Design review of the part built by this model. Coordinates are the model's own, in mm. Face numbers are marked on the shaded views. A direction names the side the tool comes from. Coordinates: 2 decimals unless noted, no trailing zeros. Loops run counter-clockwise (first coordinate to the right, second up) from the corner with the lowest first, then second, coordinate; pieces in that order, holes last.
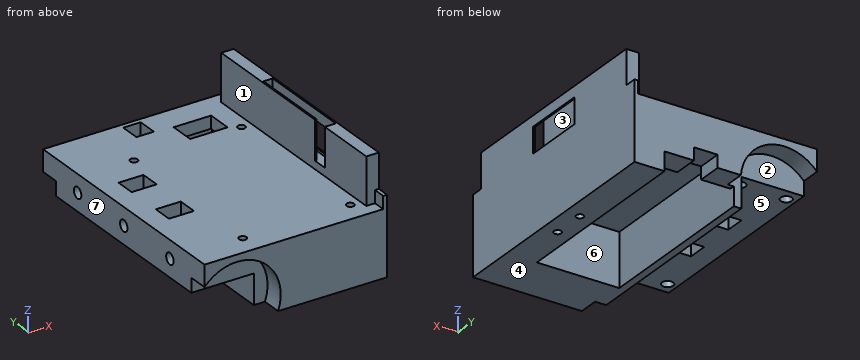
from build123d import *

# Parameters (mm, degrees)
SKETCH1_W           = 72
SKETCH1_H           = 26.25
BOSS_EXTRUDE1_DEPTH = 98
SKETCH3_W           = 24
SKETCH3_H           = 12
CUT_EXTRUDE2_DEPTH  = 98
SKETCH4_W           = 1
SKETCH4_H           = 14.25
BOSS_EXTRUDE2_DEPTH = 98
SKETCH8_R           = 17.5
CUT_EXTRUDE6_DEPTH  = 8
CUT_EXTRUDE7_START  = -8
SKETCH9_R           = 17.5
CUT_EXTRUDE7_DEPTH  = 8
SKETCH10_R          = 2.25
CUT_EXTRUDE8_DEPTH  = 4.25
SKETCH11_W          = 33
SKETCH11_H          = 67.5
CUT_EXTRUDE9_DEPTH  = 21.25
SKETCH12_W          = 33
SKETCH12_H          = 7.5
CUT_EXTRUDE10_DEPTH = 21.25
SKETCH13_W          = 9.5
SKETCH13_H          = 10
CUT_EXTRUDE11_DEPTH = 21.25
SKETCH14_W          = 5
SKETCH14_H          = 5
CUT_EXTRUDE13_DEPTH = 101.25
SKETCH17_W          = 7
SKETCH17_H          = 8
CUT_EXTRUDE14_DEPTH = 7
SKETCH18_W          = 5.398243629
SKETCH18_H          = 5.439982626
BOSS_EXTRUDE3_DEPTH = 2
SKETCH19_W          = 15
SKETCH19_H          = 15
CUT_EXTRUDE15_DEPTH = 12
SKETCH20_W          = 15.253773686
SKETCH20_H          = 5.298590198
BOSS_EXTRUDE5_DEPTH = 5
SKETCH22_R          = 1.5
CUT_EXTRUDE16_DEPTH = 8.2
SKETCH23_W          = 10
SKETCH23_H          = 8
CUT_EXTRUDE18_DEPTH = 125.988249448
SKETCH25_R          = 2.25
CUT_EXTRUDE20_DEPTH = 6.25
SKETCH26_W          = 7
SKETCH26_H          = 8
CUT_EXTRUDE21_DEPTH = 124.057913195
SKETCH28_W          = 7.366793482
SKETCH28_H          = 8.135980894
BOSS_EXTRUDE6_DEPTH = 2
SKETCH31_R          = 1.5
CUT_EXTRUDE24_DEPTH = 3.25
SKETCH32_W          = 5
SKETCH32_H          = 98
BOSS_EXTRUDE7_DEPTH = 18.75
SKETCH34_W          = 5
SKETCH34_H          = 5
CUT_EXTRUDE27_DEPTH = 13.75
SKETCH35_W          = 3.5
SKETCH35_H          = 5
CUT_EXTRUDE28_DEPTH = 5
SKETCH37_W          = 10.25
SKETCH37_H          = 25.25
CUT_EXTRUDE29_DEPTH = 3
SKETCH36_W          = 3.65
SKETCH36_H          = 38.25
CUT_EXTRUDE30_DEPTH = 15.5
SKETCH38_W          = 0.68
SKETCH38_H          = 6
CUT_EXTRUDE31_DEPTH = 15.5


with BuildPart() as part:
    # Sketch1 → Boss-Extrude1 (new body)
    with BuildSketch(Plane(origin=(0, 0, 0), x_dir=(1, 0, 0), z_dir=(0, 1, 0))):
        with Locations((-36, -13.125)):
            Rectangle(SKETCH1_W, SKETCH1_H)
    extrude(amount=BOSS_EXTRUDE1_DEPTH)

    # Sketch3 → Cut-Extrude2 (cut)
    with BuildSketch(Plane.XZ):
        with Locations((-60, 6)):
            Rectangle(SKETCH3_W, SKETCH3_H)
    extrude(amount=-CUT_EXTRUDE2_DEPTH, mode=Mode.SUBTRACT)

    # Sketch4 → Boss-Extrude2 (add)
    with BuildSketch(Plane(origin=(0, 0, 0), x_dir=(-1, 0, 0), z_dir=(0, -1, 0))):
        with Locations((72.5, -19.125)):
            Rectangle(SKETCH4_W, SKETCH4_H)
    extrude(amount=-BOSS_EXTRUDE2_DEPTH)

    # Sketch8 → Cut-Extrude6 (cut)
    with BuildSketch(Plane.XZ):
        with Locations((-60, 6)):
            Circle(SKETCH8_R)
    extrude(amount=-CUT_EXTRUDE6_DEPTH, mode=Mode.SUBTRACT)

    # Sketch9 → Cut-Extrude7 (cut)
    with BuildSketch(Plane(origin=(0, 98, 0), x_dir=(1, 0, 0), z_dir=(0, 1, 0)).offset(CUT_EXTRUDE7_START)):
        with Locations((-60, -6)):
            Circle(SKETCH9_R)
    extrude(amount=CUT_EXTRUDE7_DEPTH, mode=Mode.SUBTRACT)

    # Sketch10 → Cut-Extrude8 (cut)
    with BuildSketch(Plane(origin=(0, 0, 12), x_dir=(-1, 0, 0), z_dir=(0, 0, -1))):
        with Locations((69.25, 85)):
            Circle(SKETCH10_R)
        with Locations((50.75, 85)):
            Circle(SKETCH10_R)
        with Locations((69.25, 13)):
            Circle(SKETCH10_R)
        with Locations((50.75, 13)):
            Circle(SKETCH10_R)
    extrude(amount=-CUT_EXTRUDE8_DEPTH, mode=Mode.SUBTRACT)

    # Sketch11 → Cut-Extrude9 (cut)
    with BuildSketch(Plane(origin=(0, 0, 0), x_dir=(-1, 0, 0), z_dir=(0, 0, -1))):
        with Locations((28.5, 54.25)):
            Rectangle(SKETCH11_W, SKETCH11_H)
    extrude(amount=-CUT_EXTRUDE9_DEPTH, mode=Mode.SUBTRACT)

    # Sketch12 → Cut-Extrude10 (cut)
    with BuildSketch(Plane(origin=(0, 98, 0), x_dir=(1, 0, 0), z_dir=(0, 1, 0))):
        with Locations((-28.5, -3.75)):
            Rectangle(SKETCH12_W, SKETCH12_H)
    extrude(amount=-CUT_EXTRUDE10_DEPTH, mode=Mode.SUBTRACT)

    # Sketch13 → Cut-Extrude11 (cut)
    with BuildSketch(Plane(origin=(0, 98, 0), x_dir=(1, 0, 0), z_dir=(0, 1, 0))):
        with Locations((-28.5, -7.5)):
            Rectangle(SKETCH13_W, SKETCH13_H)
    extrude(amount=-CUT_EXTRUDE11_DEPTH, mode=Mode.SUBTRACT)

    # Sketch14 → Cut-Extrude13 (cut)
    with BuildSketch(Plane(origin=(0, 20.5, 0), x_dir=(1, 0, 0), z_dir=(0, 1, 0))):
        with Locations((-39.5, -12)):
            Rectangle(SKETCH14_W, SKETCH14_H)
    extrude(amount=CUT_EXTRUDE13_DEPTH, mode=Mode.SUBTRACT)

    # Sketch17 → Cut-Extrude14 (cut)
    with BuildSketch(Plane(origin=(0, 0, 7.5), x_dir=(-1, 0, 0), z_dir=(0, 0, -1))):
        with Locations((38.75, 92)):
            Rectangle(SKETCH17_W, SKETCH17_H)
    extrude(amount=-CUT_EXTRUDE14_DEPTH, mode=Mode.SUBTRACT)

    # Sketch18 → Boss-Extrude3 (add)
    with BuildSketch(Plane(origin=(0, 98, 0), x_dir=(1, 0, 0), z_dir=(0, 1, 0))):
        with Locations((-39.480706385, -11.994977786)):
            Rectangle(SKETCH18_W, SKETCH18_H)
    extrude(amount=-BOSS_EXTRUDE3_DEPTH)

    # Sketch19 → Cut-Extrude15 (cut)
    with BuildSketch(Plane.XY.offset(26.25)):
        with Locations((-20.5, 79.5)):
            Rectangle(SKETCH19_W, SKETCH19_H)
    extrude(amount=-CUT_EXTRUDE15_DEPTH, mode=Mode.SUBTRACT)

    # Sketch20 → Boss-Extrude5 (add)
    with BuildSketch(Plane.XY.offset(26.25)):
        with Locations((-20.373113157, 74.350704901)):
            Rectangle(SKETCH20_W, SKETCH20_H)
    extrude(amount=-BOSS_EXTRUDE5_DEPTH)

    # Sketch22 → Cut-Extrude16 (cut)
    with BuildSketch(Plane(origin=(0, 0, 0), x_dir=(-1, 0, 0), z_dir=(0, 0, -1))):
        with Locations((6, 55.73)):
            Circle(SKETCH22_R)
        with Locations((6, 42.27)):
            Circle(SKETCH22_R)
    extrude(amount=-CUT_EXTRUDE16_DEPTH, mode=Mode.SUBTRACT)

    # Sketch23 → Cut-Extrude18 (cut, through all)
    with BuildSketch(Plane.XY.offset(26.25)):
        with Locations((-60, 37.7)):
            Rectangle(SKETCH23_W, SKETCH23_H)
        with Locations((-60, 60.3)):
            Rectangle(SKETCH23_W, SKETCH23_H)
    extrude(amount=-CUT_EXTRUDE18_DEPTH, mode=Mode.SUBTRACT)

    # Sketch25 → Cut-Extrude20 (cut)
    with BuildSketch(Plane.ZY.offset(73)):
        with Locations((19.125, 77)):
            Circle(SKETCH25_R)
        with Locations((19.125, 49)):
            Circle(SKETCH25_R)
        with Locations((19.125, 21)):
            Circle(SKETCH25_R)
    extrude(amount=-CUT_EXTRUDE20_DEPTH, mode=Mode.SUBTRACT)

    # Sketch26 → Cut-Extrude21 (cut, through all)
    with BuildSketch(Plane(origin=(0, 0, 14.5), x_dir=(-1, 0, 0), z_dir=(0, 0, -1))):
        with Locations((38.75, 92)):
            Rectangle(SKETCH26_W, SKETCH26_H)
    extrude(amount=-CUT_EXTRUDE21_DEPTH, mode=Mode.SUBTRACT)

    # Sketch28 → Boss-Extrude6 (add)
    with BuildSketch(Plane(origin=(0, 0, 7.5), x_dir=(-1, 0, 0), z_dir=(0, 0, -1))):
        with Locations((38.749742444, 92.067990447)):
            Rectangle(SKETCH28_W, SKETCH28_H)
    extrude(amount=-BOSS_EXTRUDE6_DEPTH)

    # Sketch31 → Cut-Extrude24 (cut)
    with BuildSketch(Plane.XY.offset(26.25)):
        with Locations((-52.007752906, 74.651528785)):
            Circle(SKETCH31_R)
        with Locations((-9.007752906, 74.651528785)):
            Circle(SKETCH31_R)
        with Locations((-9.007752906, 8.625682812)):
            Circle(SKETCH31_R)
        with Locations((-52.007752906, 8.625682812)):
            Circle(SKETCH31_R)
    extrude(amount=-CUT_EXTRUDE24_DEPTH, mode=Mode.SUBTRACT)

    # Sketch32 → Boss-Extrude7 (add)
    with BuildSketch(Plane.XY.offset(26.25)):
        with Locations((-2.5, 49)):
            Rectangle(SKETCH32_W, SKETCH32_H)
    extrude(amount=BOSS_EXTRUDE7_DEPTH)

    # Sketch34 → Cut-Extrude27 (cut)
    with BuildSketch(Plane.XY.offset(45)):
        with Locations((-2.5, 95.5)):
            Rectangle(SKETCH34_W, SKETCH34_H)
        with Locations((-2.5, 2.5)):
            Rectangle(SKETCH34_W, SKETCH34_H)
    extrude(amount=-CUT_EXTRUDE27_DEPTH, mode=Mode.SUBTRACT)

    # Sketch35 → Cut-Extrude28 (cut)
    with BuildSketch(Plane.XY.offset(31.25)):
        with Locations((-3.25, 95.5)):
            Rectangle(SKETCH35_W, SKETCH35_H)
        with Locations((-3.25, 2.5)):
            Rectangle(SKETCH35_W, SKETCH35_H)
    extrude(amount=-CUT_EXTRUDE28_DEPTH, mode=Mode.SUBTRACT)

    # Sketch37 → Cut-Extrude29 (cut)
    with BuildSketch(Plane(origin=(0, 0, 0), x_dir=(0, 0, -1), z_dir=(1, 0, 0))):
        with Locations((-35.625, 49)):
            Rectangle(SKETCH37_W, SKETCH37_H)
    extrude(amount=-CUT_EXTRUDE29_DEPTH, mode=Mode.SUBTRACT)

    # Sketch36 → Cut-Extrude30 (cut)
    with BuildSketch(Plane.XY.offset(45)):
        with Locations((-2.5, 49.25)):
            Rectangle(SKETCH36_W, SKETCH36_H)
    extrude(amount=-CUT_EXTRUDE30_DEPTH, mode=Mode.SUBTRACT)

    # Sketch38 → Cut-Extrude31 (cut)
    with BuildSketch(Plane.XY.offset(45)):
        with Locations((-4.665, 33.125)):
            Rectangle(SKETCH38_W, SKETCH38_H)
    extrude(amount=-CUT_EXTRUDE31_DEPTH, mode=Mode.SUBTRACT)


solid = part.part
Q1. Take a section at C-C, the plane z = 27.5. Write out the cut boundary in (x, y).
Q2. Take a section at B-B, the plane x = -16. Write out the cut boundary in (y, z).
Q3. For line 1 (Y direction, x = -52, z = 24); line 2 (Y direction, x = -6, z = 2); line 3 (X direction, y = 83, z = 11.5), list the stretches that pass through material, from the lowest coordinate up.
Q4. Take a section at A-A, the plane y = 85. Write out the cut boundary in (x, z).
Q5. Machinability: for the marked faces 5, 6 and 7, which of the approach directions +Z, -Z, +X, -X, +Y, -Y give a long, thin tool a straight path to every point of the face, cutting with its end or side? Answer none if there is none.
Q6. Take a section at D-D, the plane z = 4.5. Write out the cut boundary in (x, y).
Q7. Clearance check with flat-ended pins moving along their axes: pin 1 Ø5 at (y, z) = (69.5, 30.5) entering from -X; pin 2 Ø2 at (x, y) = (-69.5, 85) entering from -Z; pin 3 Ø1.5 at (y, z) = (94.5, 9.5) entering from -X. State where each tip first meets the part, or that it passes through.
Q8. The part is to be moulded in two halves that separate along X. For the marked faces 1, 2, 3 and 4, say which applies: pulls with the +X half, pulls with the -X half, needs draft (parallel to the pull), parting line crosses it, or undercut.
Entries:
1. outline: (-5, 5) - (-1.5, 5) - (-1.5, 0) - (0, 0) - (0, 98) - (-1.5, 98) - (-1.5, 93) - (-5, 93) - close
2. outline: (0, 0) - (20.5, 0) - (20.5, 21.25) - (77, 21.25) - (77, 26.25) - (0, 26.25) - close; (87, 21.25) - (88, 21.25) - (88, 7.5) - (98, 7.5) - (98, 26.25) - (87, 26.25) - close
3. line 1: y = 0 to 7.13, 10.13 to 73.15, 76.15 to 98
3. line 2: y = 0 to 40.77, 43.77 to 54.23, 57.23 to 98
3. line 3: x = -48 to -45, -12 to 0
4. outline: (-73, 12) - (-71.5, 12) - (-71.5, 16.25) - (-67, 16.25) - (-67, 12) - (-53, 12) - (-53, 16.25) - (-48.5, 16.25) - (-48.5, 12) - (-48, 12) - (-48, 0) - (-45, 0) - (-45, 21.25) - (-28, 21.25) - (-28, 26.25) - (-73, 26.25) - close; (-13, 21.25) - (-12, 21.25) - (-12, 0) - (0, 0) - (0, 45) - (-5, 45) - (-5, 26.25) - (-13, 26.25) - close
5. face 5: -Z, -X, +Y, -Y
5. face 6: -Z
5. face 7: +Z, -Z, -X, +Y, -Y
6. outline: (-48, 8) - (-42.56, 8) - (-42.56, 0) - (0, 0) - (0, 98) - (-12, 98) - (-12, 20.5) - (-45, 20.5) - (-45, 90) - (-48, 90) - close; hole circle Ø3 at (-6, 42.27); hole circle Ø3 at (-6, 55.73)
7. pin 1: stops at x = -5
7. pin 2: stops at z = 16.25
7. pin 3: stops at x = -43.02
8. face 1: pulls with the -X half
8. face 2: undercut
8. face 3: undercut
8. face 4: needs draft
